Source: CAD feature listing. Evaluate the final solid. Frame: model axes, mm. A direction names the side the tool comes from. Coordinates: 2 decimals unless noted, no trailing zeros. Write each loop counter-clockwise with the first axis right and the second up, starting at its lowest first coordinate (ties: lowest second). Pieces come first, ordered by that corner, then holes. Notation, with made-up numbers: (46, 76) -> (57, 76) arc R14 cw to (57, 96) -> close; hole circle Ø10 at (10.25, 38.5). An arc over 180 degrees is marked (long way). Write item = value, one per line.
from build123d import *

# Parameters (mm, degrees)
F3_DEPTH = 11.8


with BuildPart() as f1:
    # F0 (on Front) → F1 (revolve)
    with BuildSketch(Plane.XZ):
        Polygon((0, 16), (0, 17), (-10, 17), (-10, 0), (-9, 0), (-9, 4.2), (-3, 4.2), (-3, 16), align=None)
    revolve(axis=Axis((0, 0, 11.945563), (0, 0, -1)))

    # F2 (on face) → F3 (join, through all)
    with BuildSketch(Plane(origin=(0, 0, 16), x_dir=(1, 0, 0), z_dir=(0, 0, -1))):
        with BuildLine():
            Line((-2, -2.236068), (-2, 2.236068))
            ThreePointArc((-2, 2.236068), (-3, 0), (-2, -2.236068))
        make_face()
    extrude(amount=F3_DEPTH)


solid = f1.part
1) Cut plane B-B, the plane x = 0. Output: boundary loops of the cut face in (y, z), and give its area (3 significant figures).
Answer block:
outline = (-10, 0) -> (-9, 0) -> (-9, 4.2) -> (-3, 4.2) -> (-3, 16) -> (3, 16) -> (3, 4.2) -> (9, 4.2) -> (9, 0) -> (10, 0) -> (10, 17) -> (-10, 17) -> close
area = 194 mm2
2) Cut plane D-D, the plane x = -2.5. Output: boundary loops of the cut face in (y, z).
Answer block:
outline = (-9.68, 0) -> (-8.65, 0) -> (-8.65, 4.2) -> (8.65, 4.2) -> (8.65, 0) -> (9.68, 0) -> (9.68, 17) -> (-9.68, 17) -> close
3) Cut plane C-C, the plane z = 15.25. Output: boundary loops of the cut face in (x, y), and give its area (3 significant figures).
Answer block:
outline = circle Ø20 at (0, 0); hole (-2, -2.24) arc R3 ccw (long way) to (-2, 2.24) -> close
area = 289 mm2
4) Material intervals for probe 1 along Y at (x, z) = (-0.25, 4); probe 2 along Y at (x, z) = (0, 9); probe 3 along Z at (x, y) = (5.5, -1.5), sorted ascending. Write a range as [from, to].
Answer block:
probe_1 = [-10, -9], [9, 10]
probe_2 = [-10, -3], [3, 10]
probe_3 = [4.2, 17]
5) Reachability of faces 1 (the flat face through (1, 0, 16)), 2 (the flat face through (0, 0, 17)) from +Z, -Z, +X, -X, +Y, -Y: full face, straight path, thin tool, end or side. Return the list, or none.
Answer block:
face_1 = -Z
face_2 = +Z, +X, -X, +Y, -Y
6) Pull-direction query (X, two-part tool) for faces 3 (the cylindrical face through (1.172, 8.923, 2.129)), 4 (the flat face through (9, 2, 0)), 5 (the cylindrical face through (2.17, -9.76, 8.38)); classes: +X half, -X half, draft (parallel to the pull), parting line (faces both ways), or undercut.
Answer block:
face_3 = undercut
face_4 = draft
face_5 = parting line
7) First-contact query: pin 1 Ø2.5 at (x, y) = (1.5, -1.5) entering from -Z; pin 2 Ø1 at (x, z) = (7, 9.5) entering from +Y; pin 3 Ø10 at (x, z) = (-1, 9) entering from -Y; pin 4 Ø2 at (x, z) = (4, 5) entering from +Y. Flat tips, straight axial feed; report the tip coordinate or a pass-through.
Answer block:
pin_1 = 4.2
pin_2 = 7.6
pin_3 = -10
pin_4 = 9.54
8) Cut plane A-A, the plane y = 0. Output: boundary loops of the cut face in (x, z).
Answer block:
outline = (-10, 0) -> (-9, 0) -> (-9, 4.2) -> (-2, 4.2) -> (-2, 16) -> (3, 16) -> (3, 4.2) -> (9, 4.2) -> (9, 0) -> (10, 0) -> (10, 17) -> (-10, 17) -> close
